The drawing under review shows one solid part. Ordinate dimensions are in mm from its lowest x, y, z. A direction names the side the tool comes from. Round coordinates to 2 decimals unless told otherwise and drop trailing zeros. Order: outer loops, then holes, each group sorted by start corner. A loop starts at its lowest first (then second) coordinate and runs counter-clockwise, first axis right, second up. Notation, with made-up numbers: M -32,-33.5 L 23,-33.5 A6 cw 23,-27.5 Z; hole C 73,56.5 d8. An arc over 180 degrees is marked long. Answer as a JSON object with one key per item and string values. Group by question number.
1) For the marked faces 1 and 2, list the 3-axis set-ups (+Z, -Z, +X, -X, +Y, -Y) from which the entire face can be reached by the end or side of a thin tool; tool diameter is ignored.
2) The part is to be moulded in two halves that separate along Y. For the marked faces 3, 4 and 5, say which applies: +Y half, -Y half, draft (parallel to the pull), parting line (faces both ways), or undercut.
3) Insertion check: pin 1 Ø11.5 at (y, z) = (38.1, 38.1) entering from +X; pin 2 Ø20.5 at (y, z) = (54, 36.5) entering from +X. Each pin has a flat end and moves straight along its axis. Give the tip position at first contact, or say it passes through.
4) To check wall thickness, follow line 1 (Y direction, x = 38.1, z = 16); line 2 (Z direction, x = 54, y = 38.1). State the ranges of each line that lie inside material, in increasing order.
5) Consider section B-B, the plane x = 67.5. Write out the cut boundary in (y, z), then the cut area to 3 significant figures.
6) Consider section A-A, the plane y = 38.1. Write out the cut boundary in (x, z).
7) Consider section C-C, the plane z = 29. Write out the cut boundary in (x, y).
8) Consider section D-D, the plane y = 19.5. Write out the cut boundary in (x, z).
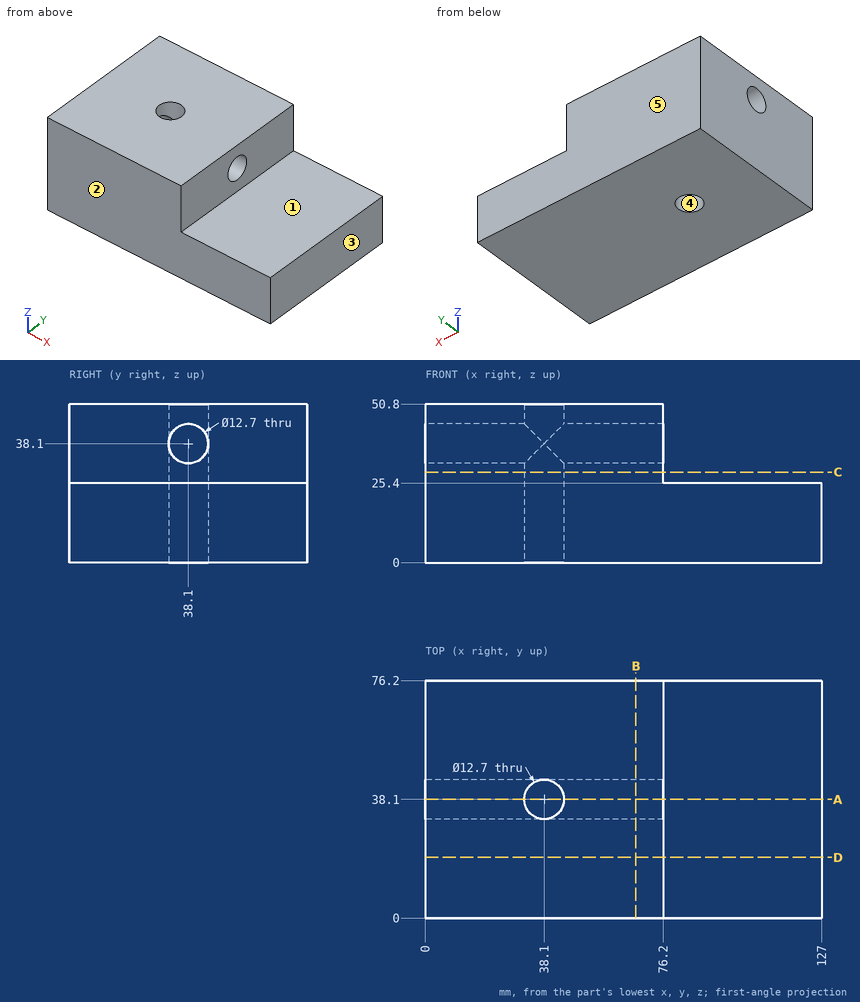
Results list:
{
 "1": {"face 1": "+Z, +X, +Y, -Y", "face 2": "+Z, -Z, +X, -X, -Y"},
 "2": {"face 3": "draft", "face 4": "undercut", "face 5": "+Y half"},
 "3": {"pin 1": "through", "pin 2": "x = 76.2"},
 "4": {"line 1": "0 to 31.75, 44.45 to 76.2", "line 2": "0 to 31.75, 44.45 to 50.8"},
 "5": {"outline": "M 0,0 L 76.2,0 L 76.2,50.8 L 0,50.8 Z; hole C 38.1,38.1 d12.7", "area": "3,740 mm^2"},
 "6": {"outline": "M 0,0 L 31.75,0 L 31.75,31.75 L 0,31.75 Z; M 0,44.45 L 31.75,44.45 L 31.75,50.8 L 0,50.8 Z; M 44.45,0 L 127,0 L 127,25.4 L 76.2,25.4 L 76.2,31.75 L 44.45,31.75 Z; M 44.45,44.45 L 76.2,44.45 L 76.2,50.8 L 44.45,50.8 Z"},
 "7": {"outline": "M 0,0 L 76.2,0 L 76.2,76.2 L 0,76.2 Z; hole C 38.1,38.1 d12.7"},
 "8": {"outline": "M 0,0 L 127,0 L 127,25.4 L 76.2,25.4 L 76.2,50.8 L 0,50.8 Z"}
}
